Geometry: final body of the model. Coordinates: model frame, mm. A direction names the side the tool comes from. Round coordinates to 2 decimals unless told otherwise and drop trailing zeros. Write each loop counter-clockwise with the first axis right and the second up, starting at its lowest first coordinate (ties: lowest second). Pieces come first, ordered by that corner, then holes. Notation, with made-up numbers: M 3.25,-5 L 53.25,-5 A12 cw 53.25,8 Z; hole C -19,18 d8. An arc over 180 degrees is marked long. Use one line per item in the form item = value. Start each with the question number.
Item 1: Pull-direction query (X, two-part tool) for faces 5 (the cylindrical face through (17.266, -2.535, 5.973)), 6 (the flat face through (-25, -4, 6.162)); classes: pulls with the +X half, pulls with the -X half, needs draft (parallel to the pull), parting line crosses it, or undercut.
Item 2: Section query D-D (x = -14). Return loops of the section in (y, z), and give its area (3 significant figures).
Item 3: Section query A-A (y = -4.3). State how many separate pieces and enclosed holes the cut face has, and give its area (3 significant figures).
Item 4: Section query C-C (z = -4.5). Return loops of the section in (x, y).
Item 5: Ray query, probe 1 along X at (y, z) = (-3.3, -1.5); probe 2 along X at (y, z) = (-3.7, 7); probe 3 along X at (y, z) = (-2.15, 3). Return the intervals inside material, ascending.
Item 6: Pin query (flat end, axial travel): pin 1 Ø2.5 at (x, y) = (24, -3.5) entering from +Z; pin 2 Ø1.5 at (x, y) = (-25.5, -3) entering from -Z; pin 3 Ø1.5 at (x, y) = (19, -1.5) entering from +Z. Return the tip coordinate at first contact, or that it passes through.
Item 7: Section query B-B (z = 15). Return loops of the section in (x, y), and give its area (3 significant figures).
Item 8: Reachability of faces 1 (the flat face through (-26, -2, 4)), 2 (the cylindrical face through (-6.07, -2.46, 13.44)), 3 (the flat face through (25, -4, 1.162)), 4 (the flat face through (-27, -3.2, 5)) from +Z, -Z, +X, -X, +Y, -Y: full face, straight path, thin tool, end or side. Return the list, or none.
from build123d import *

# Parameters (mm, degrees)
F1_DEPTH       = 5
F2_W           = 15
F2_H           = 33.127493
F3_DEPTH       = 25
F4_R           = 5
F6_DEPTH       = 3
F7_D           = 2.2
F7_DEPTH       = 40
F7_CBORE_D     = 4.4
F7_CBORE_DEPTH = 1.8
F8_R           = 2
F9_DEPTH       = 25


with BuildPart() as f1:
    # F0 (on Front) → F1 (new body)
    with BuildSketch(Plane.XZ):
        with BuildLine():
            Line((-22.5, -17.5), (22.5, -17.5))
            Line((22.5, -17.5), (22.5, 17.5))
            ThreePointArc((22.5, 17.5), (0, 28.504386), (-22.5, 17.5))
            Line((-22.5, 17.5), (-22.5, -17.5))
        make_face()
    extrude(amount=F1_DEPTH)

    # F2 (on face) → F3 (cut)
    with BuildSketch(Plane.XZ.offset(5)):
        with Locations((0, 28.504385)):
            Rectangle(F2_W, F2_H)
    extrude(amount=-F3_DEPTH, mode=Mode.SUBTRACT)

    # F4
    f4_edges = [f1.edges().sort_by_distance(p)[0] for p in [
        (-7.5, -2.5, 11.940639),
        (7.5, -2.5, 11.940639),
    ]]
    fillet(f4_edges, radius=F4_R)

    # F5 (on face) → F6 (join)
    with BuildSketch(Plane.XZ.offset(5)):
        with BuildLine():
            Line((-22.5, 1.162), (-22.5, 6.162))
            Line((-22.5, 6.162), (-27.5, 6.162))
            ThreePointArc((-27.5, 6.162), (-30, 3.662), (-27.5, 1.162))
            Line((-27.5, 1.162), (-22.5, 1.162))
        make_face()
        with BuildLine():
            Line((22.5, 1.162), (27.5, 1.162))
            ThreePointArc((27.5, 1.162), (30, 3.662), (27.5, 6.162))
            Line((27.5, 6.162), (22.5, 6.162))
            Line((22.5, 6.162), (22.5, 1.162))
        make_face()
    extrude(amount=-F6_DEPTH)

    # F7
    with Locations(Plane.XZ.offset(5)):
        with Locations((-27.5, 3.662), (27.5, 3.662)):
            CounterBoreHole(F7_D / 2, F7_CBORE_D / 2, F7_CBORE_DEPTH, depth=F7_DEPTH)

    # F8 (on face) → F9 (cut)
    with BuildSketch(Plane.XZ.offset(5)):
        with Locations((-17.581366, -13.26084)):
            Circle(F8_R)
        with Locations((-17.581366, -3.26084)):
            Circle(F8_R)
        with Locations((-17.581366, 6.73916)):
            Circle(F8_R)
        with Locations((-6.581366, -13.26084)):
            Circle(F8_R)
        with Locations((-6.581366, -3.26084)):
            Circle(F8_R)
        with Locations((-6.581366, 6.73916)):
            Circle(F8_R)
        with Locations((4.418634, -13.26084)):
            Circle(F8_R)
        with Locations((4.418634, -3.26084)):
            Circle(F8_R)
        with Locations((4.418634, 6.73916)):
            Circle(F8_R)
        with Locations((15.418634, -13.26084)):
            Circle(F8_R)
        with Locations((15.418634, -3.26084)):
            Circle(F8_R)
        with Locations((15.418634, 6.73916)):
            Circle(F8_R)
    extrude(amount=-F9_DEPTH, mode=Mode.SUBTRACT)


solid = f1.part
Working result:
q1.face_5 = undercut
q1.face_6 = needs draft
q2.outline = M -5,-17.5 L 0,-17.5 L 0,24.83 L -5,24.83 Z
q2.area = 212 mm²
q3.separate_pieces = 1
q3.enclosed_holes = 14
q3.area = 1,580 mm²
q4.outline = M -22.5,-5 L -19.15,-5 L -19.15,0 L -22.5,0 Z; M -16.01,-5 L -8.15,-5 L -8.15,0 L -16.01,0 Z; M -5.01,-5 L 2.85,-5 L 2.85,0 L -5.01,0 Z; M 5.99,-5 L 13.85,-5 L 13.85,0 L 5.99,0 Z; M 16.99,-5 L 22.5,-5 L 22.5,0 L 16.99,0 Z
q5.probe_1 = -22.5 to -18.53, -16.63 to -7.53, -5.63 to 3.47, 5.37 to 14.47, 16.37 to 22.5
q5.probe_2 = -22.5 to -19.56, -15.6 to -8.56, -4.6 to 2.44, 6.4 to 13.44, 17.4 to 22.5
q5.probe_3 = -29.91 to -28.38, -26.62 to 26.62, 28.38 to 29.91
q6.pin_1 = 6.16
q6.pin_2 = 1.16
q6.pin_3 = 21.9
q7.outline = M -22.5,-5 L -7.11,-5 L -7.11,0 L -22.5,0 Z; M 7.11,-5 L 22.5,-5 L 22.5,0 L 7.11,0 Z
q7.area = 154 mm²
q8.face_1 = +Z, -Z, -X, +Y
q8.face_2 = +Z, +Y, -Y
q8.face_3 = -Z, +X, +Y, -Y
q8.face_4 = -Y
